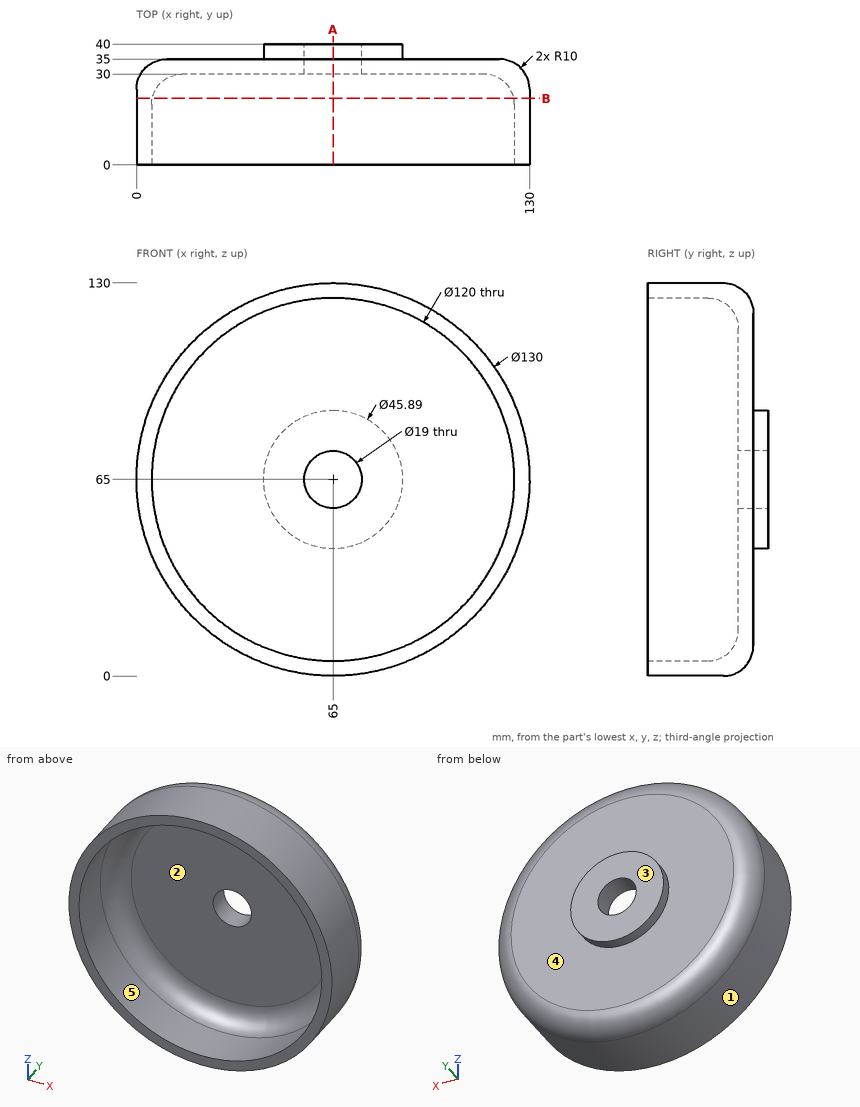
Design review of the part shown in the three views and the two pictorial views. Dimensions are in mm from the part's minimum x, y and z. A direction names the side the tool comes from. Give positions to 0.01 mm unless a question says otherwise; leave off trailing zeros. Write each loop counter-clockwise with the first axis right and the second up, starting at its lowest first coordinate (ties: lowest second). Pieces come first, ordered by that corner, then holes.
Item 1: Wall thickness on probe 1 along X at (y, z) = (5.25, 65); probe 2 along Z at (x, y) = (63.5, 7); probe 3 along X at (y, z) = (35.75, 65) (3 decimals): over which ranges is each line inside the solid? List them lowest first.
Item 2: Take a section at B-B (y = 22). Give the boundary of the cut face in (x, z), and give its area (3 significant figures).
Item 3: Insertion check: P1, Ø8, axis at x = 51.5, y = 26.5, coming from the -Z side; P2, Ø8, axis at x = 66.5, z = 103.5, coming from the -Y side; P3, Ø12, axis at x = 48, z = 38.5, coming from the +Y side. Each pin has a flat end and moves straight along its axis. Give the tip position at first contact, or say it passes through.
Item 4: The part is to be moulded in two halves that separate along X. For the marked faces 1, 2 and 3, say which applies: +X half, -X half, draft (parallel to the pull), parting line (faces both ways), or undercut.
Item 5: Machinability: for the marked faces 4 and 5, which of the approach directions +Z, -Z, +X, -X, +Y, -Y give a long, thin tool a straight path to every point of the face, cutting with its end or side? Answer none if there is none.
Item 6: Take a section at A-A (x = 65). Give the boundary of the cut face in (y, z) (3 decimals), and give its area (3 significant figures).
Established:
1. probe 1: x = 0 to 5, 125 to 130
1. probe 2: z = 0.02 to 5.02, 124.98 to 129.98
1. probe 3: x = 42.055 to 55.5, 74.5 to 87.945
2. outline: circle Ø130 at (65, 65); hole circle Ø119.6 at (65, 65)
2. area: 2,040 mm2
3. P1: stops at z = 0.73
3. P2: stops at y = 30
3. P3: stops at y = 35
4. face 1: parting line
4. face 2: undercut
4. face 3: draft
5. face 4: +Y
5. face 5: -Y
6. outline: (0, 0) - (25, 0) arc R10 ccw to (35, 10) - (35, 42.055) - (40, 42.055) - (40, 55.5) - (30, 55.5) - (30, 15) arc R10 cw to (20, 5) - (0, 5) - close; (0, 125) - (20, 125) arc R10 cw to (30, 115) - (30, 74.5) - (40, 74.5) - (40, 87.945) - (35, 87.945) - (35, 120) arc R10 ccw to (25, 130) - (0, 130) - close
6. area: 989 mm2
